Verification items for the finished model (mm, model axes). Face numbers are marked on the shaded views. A direction names the side the tool comes from. Give positions to 0.01 mm unless a question says otherwise; leave off trailing zeros. Loops run counter-clockwise (first coordinate to the right, second up) from the corner with the lowest first, then second, coordinate; pieces in that order, holes last. Notation, with made-up numbers: (-1, 44.25) - (44, 44.25) arc R26 cw to (44, 67.25) - close; hole circle Ø7 at (76.25, -3.5). An arc over 180 degrees is marked (long way). One line per item, written item: value. Start each with the question number.
1. Sectioned sample at B-B (y = 52). Record the cut outline in (x, z), plus the area to 3 significant figures.
2. Mould release check, pull along Y, two halves, no side actions. Record for the marked faces 1, 2 and 3: pulls with the +Y half, pulls with the -Y half, needs draft (parallel to the pull), parting line crosses it, or undercut.
3. Access from +Z, -Z, +X, -X, +Y, -Y to the whole of each face (thin tool, end or side, straight path). Record for the marked faces 4 and 5.
4. Sectioned sample at A-A (z = 53.5). Count the separate pieces of the cut face and the enclosed holes in it, plus the area to 3 significant figures.
5. Sectioned sample at D-D (y = 108). Record the cut outline in (x, z).
6. Scan lines: L1, parallel to X at y = 193, z = -2.5; L2, parallel to X at y = 130, z = -1; L3, parallel to Y at x = -18.5, z = 4. Record each from-to range of solid material in increasing order. Write a range as [from, to].
7. Gauge pin test, flat ends, axial feed: pin 1 (1.5 mm diameter, centred on y = 81, z = 36, fed in from +X); pin 2 (1 mm diameter, centred on x = 23, y = 86.5, fed in from +Z); pin 3 (2 mm diameter, centred on y = 109.5, z = -44, fed in from -X). Record the tip position at first contact, or that the pin passes through.
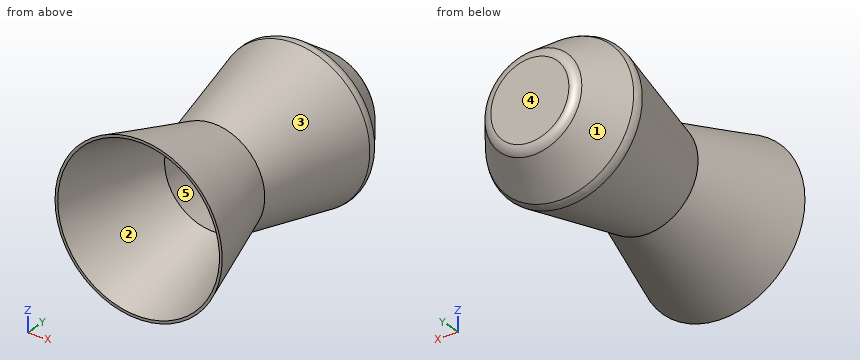
Autodesk Fusion 360 part; units mm, degrees
sketch "Esquisse1" plane through (0, 0, 0) normal (0, 0, 1) x (1, 0, 0)
  line L0 (0, 0) -> (-65, 0)
  line L1 (-65, 0) -> (-40, 80)
  line L2 (-40, 80) -> (-60, 170)
  line L3 (-60, 170) -> (-35, 205)
  line L4 (-35, 205) -> (0, 205)
  line L5 (0, 205) -> (0, 0)
  dimension "d1" = 65
  dimension "d3" = 35
  dimension "d4" = 90
  dimension "d5" = 80
  dimension "d6" = 40
  dimension "d7" = 60
  dimension "d8" = 35
revolve "Révolution1" add sketch "Esquisse1" angle 360 about axis through (0, 205, 0) along (0, -1, 0)
fillet "Congé1" radius 9 1 edges at (-55.9396, 170, 21.6969)
fillet "Congé2" radius 9 1 edges at (-32.6315, 205, 12.6565)
shell "Coque1" thickness 2 removed faces 1 at (20.2416, 0, -0.2148)
Results are:
1. outline: circle Ø97.5 at (0, 0); hole circle Ø93.31 at (0, 0)
1. area: 628 mm^2
2. face 1: pulls with the +Y half
2. face 2: pulls with the -Y half
2. face 3: undercut
3. face 4: +Z, -Z, +X, -X, +Y
3. face 5: none
4. separate pieces: 2
4. enclosed holes: 1
4. area: 1,090 mm^2
5. outline: circle Ø92.44 at (0, 0); hole circle Ø88.35 at (0, 0)
6. L1: x = [-43.5, -41.04], [41.04, 43.5]
6. L2: x = [-51.1, -49.05], [49.05, 51.1]
6. L3: y = [203, 205]
7. pin 1: stops at x = 19.41
7. pin 2: stops at z = 34.83
7. pin 3: stops at x = -17.91
